Autodesk Inventor part; units mm, degrees
ref_plane "YZ Plane" through (0, 0, 0) normal (1, 0, 0) x (0, 1, 0)
ref_plane "XZ Plane" through (0, 0, 0) normal (0, 1, 0) x (-1, 0, 0)
ref_plane "XY Plane" through (0, 0, 0) normal (0, 0, 1) x (1, 0, 0)
sketch "Sketch1" plane through (0, 0, 0) normal (0, 1, 0) x (-1, 0, 0)
  circle A0 centre (-9.9449, -17.225) radius 1 construction
  circle A1 centre (8.4149, -17.225) radius 1 construction
  circle A2 centre (22.1847, 17.225) radius 1 construction
  circle A3 centre (-23.7147, 17.225) radius 1 construction
  circle A4 centre (-9.9449, -17.225) radius 2
  circle A5 centre (8.4149, -17.225) radius 2
  circle A6 centre (22.1847, 17.225) radius 2
  circle A7 centre (-23.7147, 17.225) radius 2
  line L0 (30, -25) -> (-30, -25)
  line L1 (-30, -25) -> (-30, 25)
  line L2 (-30, 25) -> (30, 25)
  line L3 (30, 25) -> (30, -25)
  line L4 (0, -35) -> (0, 35)
  line L5 (42, 0) -> (-42, 0)
  point P0 (0, 0)
  point P1 (25.2446, -19.875)
  dimension "d0" = 25.2446
  dimension "d1" = 19.875
  dimension "d2" = 16.8298
  dimension "d3" = 18.3597
  dimension "d4" = 2.65
  dimension "d5" = 37.1
  dimension "d6" = 3.06
  dimension "d7" = 45.8993
  dimension "d9" = 2
  dimension "d10" = 1
  dimension "d11" = 60
  dimension "d12" = 50
extrude "Extrusion1" add sketch "Sketch1" along normal blind 5 contours A4 | A5 | A6 | A7
extrude "Extrusion2" add sketch "Sketch1" along normal blind 2
chamfer "Chamfer1" distance 2.5 angle 45 4 edges at (-6.4149, 2, -17.225) (11.9449, 2, -17.225) (25.7147, 2, 17.225) (-20.1847, 2, 17.225)
hole "Hole1" at (-8.4149, 0, -17.225) at (9.9449, 0, -17.225) at (-22.1847, 0, 17.225) at (23.7147, 0, 17.225) direction (0, 1, 0) diameter 2.2 end through all counterbore diameter 4.4 counterbore depth 1.6
equation "\"pitch\" = 5.3"
equation "\"pitch_x\" = 0.866025 * pitch"
equation "\"cell_w\" = 1.1547 * pitch"
properties part number "Panel mount plate"
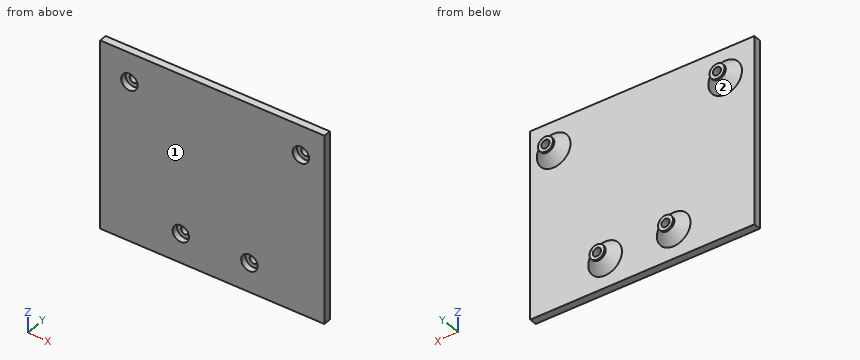
For this review, take the finished solid that the model builds, in its own axes (mm). Face numbers are marked on the shaded views. Round coordinates to 2 decimals unless told otherwise and drop trailing zeros. Loops run counter-clockwise (first coordinate to the right, second up) from the corner with the lowest first, then second, coordinate; pieces in that order, holes last. Notation, with made-up numbers: (-25.75, 4.25) - (6.25, 4.25) arc R24 ccw to (6.25, 19.25) - close; hole circle Ø10 at (-18.75, 4). An arc over 180 degrees is marked (long way). One line per question, with ' | ' between items.
Q1. Take a section at B-B (z = 6). Give the boundary of the cut face in (x, y), and give its area (3 significant figures).
Taken from the geometry:
outline: (-30, 0) - (30, 0) - (30, 2) - (-30, 2) - close | area: 120 mm²
Q2. Take a section at A-A (y = 3.25). Give the boundary of the cut face in (x, z) (3 decimals), and give its area (3 significant figures).
Taken from the geometry:
outline: circle Ø6.5 at (-22.185, 17.225); circle Ø6.5 at (-8.415, -17.225); circle Ø6.5 at (9.945, -17.225); circle Ø6.5 at (23.715, 17.225); hole circle Ø2.2 at (-22.185, 17.225); hole circle Ø2.2 at (-8.415, -17.225); hole circle Ø2.2 at (9.945, -17.225); hole circle Ø2.2 at (23.715, 17.225) | area: 118 mm²
Q3. Take a section at C-C (x = 0.5). Give the boundary of the cut face in (y, z), and give its area (3 significant figures).
Taken from the geometry:
outline: (0, -25) - (2, -25) - (2, 25) - (0, 25) - close | area: 100 mm²
Q4. For pin 1 (1.8 mm diameter, centred on x = 9.94, z = -17.23, fed in from +Y); pin 2 (4 mm diameter, centred on x = 4, z = 13, fed in from +Y); pin 3 (2.5 mm diameter, centred on x = -8.41, z = -17.23, fed in from -Y), all flat-tipped, find the tip position at first contact; note any pin that passes through.
Taken from the geometry:
pin 1: passes through | pin 2: stops at y = 2 | pin 3: stops at y = 1.6
Q5. For line 1 along Z through (x, y) = (-22, 0.4); line 2 along X through (y, z) = (2.9, 18); line 3 along X through (y, z) = (1.15, 16), list the stretches that pass through material, from the lowest coordinate up. Write a range as [from, to].
Taken from the geometry:
line 1: z = [-25, 15.03], [19.42, 25] | line 2: x = [-25.7, -22.97], [-21.4, -18.67], [20.2, 22.93], [24.5, 27.23] | line 3: x = [-30, -24.01], [-20.36, 21.89], [25.54, 30]
Q6. The part is to be moulded in two halves that separate along X. For the marked faces 1 and 2, say which applies: released by +X, released by -X, zero draft, split by the parting line, or undercut.
Taken from the geometry:
face 1: zero draft | face 2: undercut
